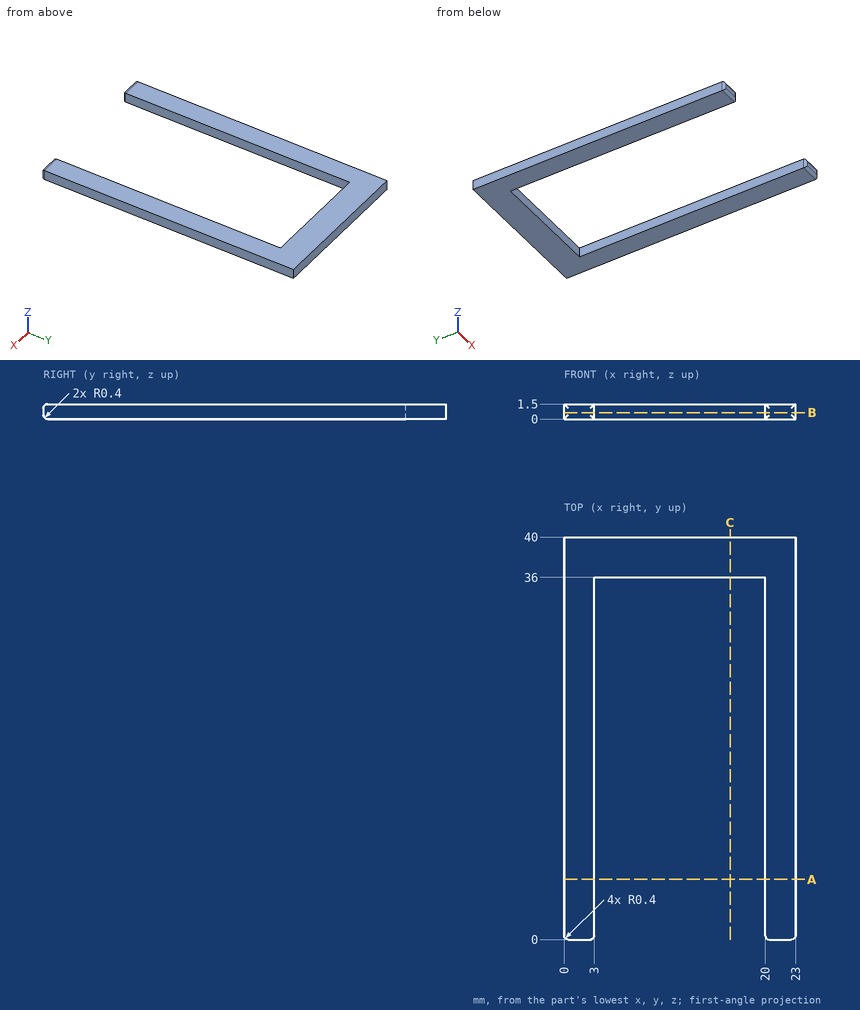
Check sheet for the drawn part. Datum: minimum x, y, z corner. Units: mm. Round coordinates to 2 decimals unless told otherwise and drop trailing zeros. Loops run counter-clockwise (first coordinate to the right, second up) from the corner with the lowest first, then second, coordinate; pieces in that order, holes last. Notation, with made-up numbers: (48.5, -12.5) -> (103.5, -12.5) arc R21 ccw to (103.5, -4.5) -> close; hole circle Ø5 at (43, 12). An arc over 180 degrees is marked (long way). Put each result on its own line as item: value. Start each with the question number.
1. Section check A-A (y = 6). Enter the section's corners in (x, z), plus the area to 3 significant figures.
2. Section check C-C (x = 16.5). Enter the section's corners in (y, z).
3. Scan lines: probe 1 along X at (y, z) = (10.5, 0.3); probe 2 along Y at (x, z) = (4, 0.3). Record each from-to range of solid material in increasing order.
4. Section check B-B (z = 0.65). Enter the section's corners in (x, y).
Findings:
1. outline: (0, 0) -> (3, 0) -> (3, 1.5) -> (0, 1.5) -> close; (20, 0) -> (23, 0) -> (23, 1.5) -> (20, 1.5) -> close
1. area: 9.00 mm^2
2. outline: (36, 0) -> (40, 0) -> (40, 1.5) -> (36, 1.5) -> close
3. probe 1: x = 0 to 3, 20 to 23
3. probe 2: y = 36 to 40
4. outline: (0, 0.4) arc R0.4 ccw to (0.4, 0) -> (2.6, 0) arc R0.4 ccw to (3, 0.4) -> (3, 36) -> (20, 36) -> (20, 0.4) arc R0.4 ccw to (20.4, 0) -> (22.6, 0) arc R0.4 ccw to (23, 0.4) -> (23, 40) -> (0, 40) -> close
